```python
from build123d import *

# Parameters (mm, degrees)
SKETCH13_R              = 1.651
BASE_FLANGE5_DEPTH      = 3.175
EDGE_FLANGE4_START      = -48.484504913
EDGE_FLANGE4_DEPTH      = 25.4
CUT_EXTRUDE4_DEPTH      = 34.925
CUT_EXTRUDE4_DEPTH_BACK = 5.588


# Read off the part's stored shape, not the designer's step: Edge-Flange4
# Sheet-metal steps are written as plain solids
with BuildPart() as part:
    # Sketch13 → Base-Flange5 (new body)
    with BuildSketch(Plane.XY):
        Polygon((-66.04, 0), (0, 0), (0, -23.797677877), (-74.918655736, -23.797677877), align=None)
        with Locations((-7.112, -12.296727665)):
            Circle(SKETCH13_R, mode=Mode.SUBTRACT)
    extrude(amount=-BASE_FLANGE5_DEPTH)

    # Edge-Flange4 outline → Edge-Flange4 (add)
    with BuildSketch(Plane(origin=(0, 0, 0), x_dir=(0.9369164518419233, -0.34955337542060905, 0), z_dir=(0.34955337542060905, 0.9369164518419232, 0)).offset(EDGE_FLANGE4_START)):
        with BuildLine():
            Line((-61.87396248, -28.575), (-61.87396248, 3.175))
            ThreePointArc((-61.87396248, 3.175), (-64.11902651, 2.24506403), (-65.04896248, 0))
            Line((-65.04896248, 0), (-65.04896248, -28.575))
            Line((-65.04896248, -28.575), (-61.87396248, -28.575))
        make_face()
    extrude(amount=EDGE_FLANGE4_DEPTH)

    # Sketch51 → Cut-Extrude4 (cut, two sides: drawn at the far end of the back side and taken through both)
    with BuildSketch(Plane.XY.offset(-CUT_EXTRUDE4_DEPTH_BACK)):
        Polygon((-66.04, 0), (-69.428776015, 0), (-69.014709735, 1.109831967), align=None)
    extrude(amount=CUT_EXTRUDE4_DEPTH + CUT_EXTRUDE4_DEPTH_BACK, mode=Mode.SUBTRACT)


solid = part.part
```
The model under review builds one solid part; all positions refer to its coordinate system, in mm. Round coordinates to 2 decimals unless told otherwise and drop trailing zeros. Loops run counter-clockwise (first coordinate to the right, second up) from the corner with the lowest first, then second, coordinate; pieces in that order, holes last. Notation, with made-up numbers: (-34, -25) - (-21, -25) arc R14 ccw to (-21, -10) - close; hole circle Ø4 at (68, 76.5). An arc over 180 degrees is marked (long way). Write each question's results on one line, items separated by ' | '. Start each with the question number.
Q1. Insertion check: P1, Ø4, axis at x = -7.11, y = -12.3, coming from the -Z side (3 decimals); P2, Ø5, axis at y = -15, z = 9.5, coming from the +X side; P3, Ø1.5, axis at y = -7, z = 2, coming from the +X side. Each pin has a flat end and moves straight along its axis. Give the tip position at first contact, or say it passes through.
Q2. Wall thickness on line 1 along Z through (x, y) = (-13, -1.75) (3 decimals); line 2 along X through (y, z) = (-8, 27); line 3 along X through (y, z) = (-10, -0.5): over which ranges is each line inside the solid? List them lowest first. Write a range as [from, to].
Q3. Draft analysis for pull direction Y (two halves, no side actions). For faces 1 (the flat face through (-70.541, -12.065, 14.488)), 2 (the flat face through (-37, -12, 0)), 3 (the cylindrical face through (-8.422, -13.301, -1.565)), 4 (the cylindrical face through (-72.62, -11.29, -2.27)), state which applies: pulls with the +Y half, pulls with the -Y half, needs draft (parallel to the pull), parting line crosses it, or undercut.
Q4. Take a section at B-B on x = -42. Give the boundary of the cut face in (y, z) (3 decimals).
Q5. Take a section at A-A on z = 17.5. Give the boundary of the cut face in (x, y), plus the area to 3 significant figures.
Data:
1) P1: stops at z = -3.175 | P2: stops at x = -70.7 | P3: stops at x = -68.37
2) line 1: z = [-3.175, 0] | line 2: x = [-72.41, -69.02] | line 3: x = [-73.12, 0]
3) face 1: pulls with the -Y half | face 2: needs draft | face 3: undercut | face 4: pulls with the +Y half
4) outline: (-23.798, -3.175) - (0, -3.175) - (0, 0) - (-23.798, 0) - close
5) outline: (-77.89, -22.69) - (-74.92, -23.8) - (-66.04, 0) - (-69.43, 0) - close | area: 78.8 mm²
